Autodesk Inventor part; units mm, degrees
ref_plane "YZ Plane" through (0, 0, 0) normal (1, 0, 0) x (0, 1, 0)
ref_plane "XZ Plane" through (0, 0, 0) normal (0, 1, 0) x (-1, 0, 0)
ref_plane "XY Plane" through (0, 0, 0) normal (0, 0, 1) x (1, 0, 0)
sketch "Sketch1" plane through (0, 0, 0) normal (0, 0, 1) x (1, 0, 0)
  circle A0 centre (0, 0) radius 15.5
  line L0 (-20, 0) -> (20, 0) construction
  line L1 (-20, -4) -> (20, -4)
  line L2 (20, 4) -> (-20, 4)
  arc A1 (-20, 4) -> (-20, -4) centre (-20, 0) ccw
  arc A2 (20, -4) -> (20, 4) centre (20, 0) ccw
  line L3 (0, -20) -> (0, 20) construction
  line L4 (4, -20) -> (4, 20)
  line L5 (-4, 20) -> (-4, -20)
  arc A3 (-4, -20) -> (4, -20) centre (0, -20) ccw
  arc A4 (4, 20) -> (-4, 20) centre (0, 20) ccw
  circle A5 centre (-20, 0) radius 1.75
  circle A6 centre (0, 20) radius 1.75
  circle A7 centre (20, 0) radius 1.75
  circle A8 centre (0, -20) radius 1.75
  point P0 (4, -14.975)
  point P1 (14.975, -4)
  point P2 (14.975, 4)
  point P3 (4, 14.975)
  point P4 (-4, 14.975)
  point P5 (-14.975, 4)
  point P6 (-14.975, -4)
  point P7 (-4, -14.975)
  dimension "d0" = 40
  dimension "d1" = 40
  dimension "d2" = 4
  dimension "d3" = 4
  dimension "d4" = 31
  dimension "d5" = 3.5
extrude "Extrusion1" add sketch "Sketch1" along normal blind 1
chamfer "Chamfer1" distance 0.5 angle 45 16 edges at (-10.9602, -10.9602, 0) (-4, -17.4875, 0) (0, -24, 0) (4, -17.4875, 0) (10.9602, -10.9602, 0) (17.4875, -4, 0) (24, 0, 0) (17.4875, 4, 0) (10.9602, 10.9602, 0) (4, 17.4875, 0) (0, 24, 0) (-4, 17.4875, 0) (-10.9602, 10.9602, 0) (-17.4875, 4, 0) (-24, 0, 0) (-17.4875, -4, 0)
properties part number "PlatformBracket"
Geometry check sheet. Reference: the model listing, model coordinates, mm. Round coordinates to 2 decimals unless told otherwise and drop trailing zeros. Write each loop counter-clockwise with the first axis right and the second up, starting at its lowest first coordinate (ties: lowest second). Pieces come first, ordered by that corner, then holes. Notation, with made-up numbers: (-3, -7) -> (11, -7) arc R4 ccw to (11, 0) -> close; hole circle Ø4 at (34.25, 85.25). An arc over 180 degrees is marked (long way). One line per item, written item: value. Start each with the question number.
(1) Go/stop test with flat-tipped pins: pin 1 Ø4.5 at (x, y) = (-20, 0) entering from -Z; pin 2 Ø0.6 at (x, z) = (-18.5, 0.5) entering from -Y; pin 3 Ø0.6 at (y, z) = (-18.5, 0.5) entering from -X; pin 4 Ø0.6 at (y, z) = (17, 1) entering from +X. Record where each tip stops, or that it passes through.
(2) Cross-section at C-C, the plane z = 0.3. Record the cut outline in (x, y), and give its area (3 significant figures).
(3) Cross-section at D-D, the plane x = 16. Record the cut outline in (y, z), and give its area (3 significant figures).
(4) Draft check along Y on faces 1 (the cylindrical face through (-0.1, 24, 0.7)), 2 (the cylindrical face through (-10.88, -11.04, 0.75)), 3 (the cylindrical face through (-0.228, -21.735, 0.493)). Enter one of: +Y half, -Y half, draft (parallel to the pull), parting line (faces both ways), or undercut.
(5) Scan lines: line 1 (Y direction, x = 20, z = 0.7); line 2 (Y direction, x = 0, z = 0.3); line 3 (Y direction, x = 0, z = 0.6). Record each from-to range of solid material in increasing order. Write a range as [from, to].
(6) Cross-section at A-A, the plane y = 0. Record the cut outline in (x, z), and give its area (4 significant figures).
Answer:
1. pin 1: z = 0
1. pin 2: y = -4
1. pin 3: x = -4
1. pin 4: x = 4
2. outline: (-20, -3.8) -> (-14.82, -3.8) arc R15.3 ccw to (-3.8, -14.82) -> (-3.8, -20) arc R3.8 ccw to (3.8, -20) -> (3.8, -14.82) arc R15.3 ccw to (14.82, -3.8) -> (20, -3.8) arc R3.8 ccw to (20, 3.8) -> (14.82, 3.8) arc R15.3 ccw to (3.8, 14.82) -> (3.8, 20) arc R3.8 ccw to (-3.8, 20) -> (-3.8, 14.82) arc R15.3 ccw to (-14.82, 3.8) -> (-20, 3.8) arc R3.8 ccw to start; hole circle Ø3.5 at (-20, 0); hole circle Ø3.5 at (0, -20); hole circle Ø3.5 at (0, 20); hole circle Ø3.5 at (20, 0)
2. area: 935 mm²
3. outline: (-4, 0.5) -> (-3.5, 0) -> (3.5, 0) -> (4, 0.5) -> (4, 1) -> (-4, 1) -> close
3. area: 7.75 mm²
4. face 1: +Y half
4. face 2: -Y half
4. face 3: undercut
5. line 1: [-4, -1.75], [1.75, 4]
5. line 2: [-23.8, -21.75], [-18.25, 18.25], [21.75, 23.8]
5. line 3: [-24, -21.75], [-18.25, 18.25], [21.75, 24]
6. outline: (-24, 0.5) -> (-23.5, 0) -> (-21.75, 0) -> (-21.75, 1) -> (-24, 1) -> close; (-18.25, 0) -> (18.25, 0) -> (18.25, 1) -> (-18.25, 1) -> close; (21.75, 0) -> (23.5, 0) -> (24, 0.5) -> (24, 1) -> (21.75, 1) -> close
6. area: 40.75 mm²
